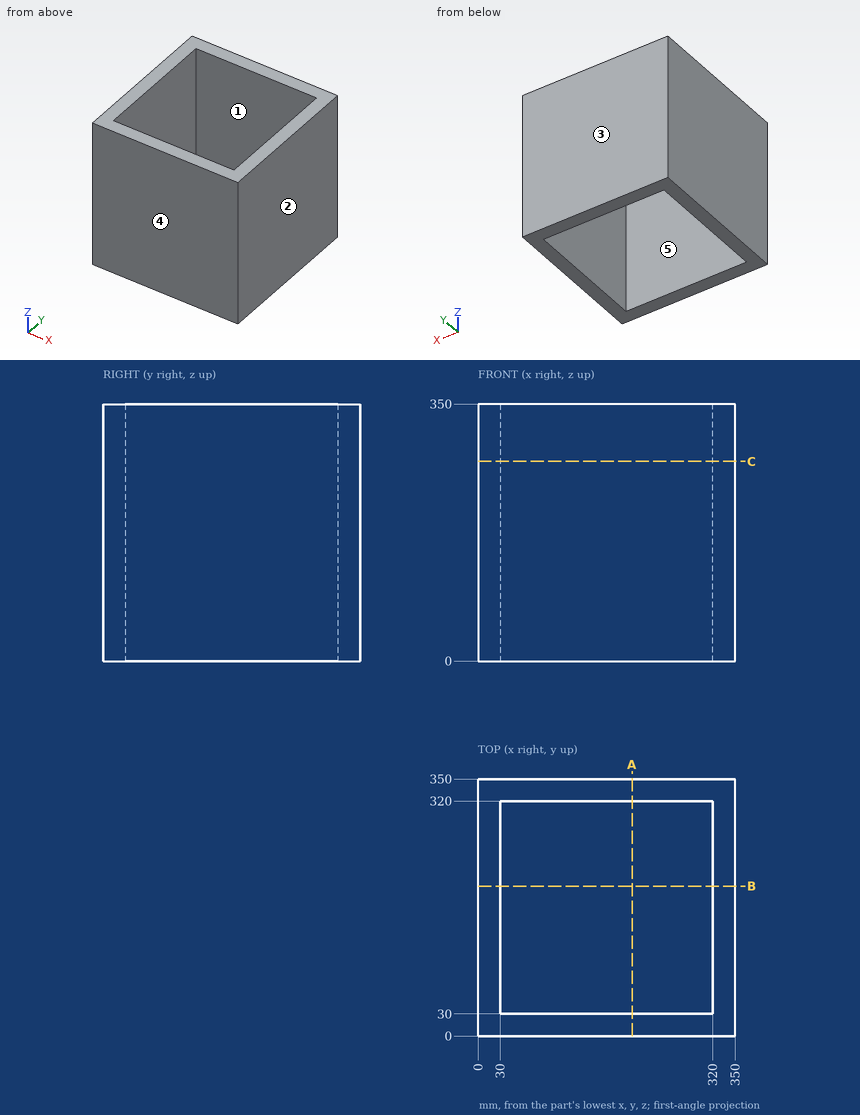
Geometry check sheet. Reference: drawing and pictorial views, mm from the part's lowest x, y, z. A direction names the side the tool comes from. Round coordinates to 2 decimals unless told otherwise and drop trailing zeros. Loops run counter-clockwise (first coordinate to the right, second up) from the corner with the lowest first, then second, coordinate; pieces in that order, holes last. Notation, with made-up numbers: (-7, -3) -> (3, -3) arc R12 cw to (3, 16) -> close; hole circle Ø5 at (68, 25.5). An arc over 180 degrees is marked (long way). Answer as a JSON object with one key per item and string values. Group by question number.
Item 1: Set-up check for the marked faces 4 and 5: record each of +Z, -Z, +X, -X, +Y, -Y from which the full face is reachable in a straight line by a thin tool's end or side.
Item 2: Cross-section at C-C, the plane z = 272. Record the cut outline in (x, y), plus the area to 3 significant figures.
Item 3: Release check for a two-part mould opening along X. For the marked faces 1, 2 and 3 record: pulls with the +X half, pulls with the -X half, needs draft (parallel to the pull), parting line crosses it, or undercut.
Item 4: Thickness scan on line 1 along Y through (x, z) = (242, 178.5). Record the ranges inside material, lowest first.
Item 5: Depth check by flat-ended pin: pin 1 Ø3 at (x, z) = (305.5, 156.5) entering from -Y. Enter the tip coordinate at first touch or a pass-through.
Item 6: Cross-section at A-A, the plane x = 210. Record the cut outline in (y, z), plus the area to 3 significant figures.
Determined:
{
 "1": {"face 4": "+Z, -Z, +X, -X, -Y", "face 5": "+Z, -Z"},
 "2": {"outline": "(0, 0) -> (350, 0) -> (350, 350) -> (0, 350) -> close; hole (30, 30) -> (320, 30) -> (320, 320) -> (30, 320) -> close", "area": "38,400 mm²"},
 "3": {"face 1": "undercut", "face 2": "pulls with the +X half", "face 3": "needs draft"},
 "4": {"line 1": "y = 0 to 30, 320 to 350"},
 "5": {"pin 1": "stops at y = 0"},
 "6": {"outline": "(0, 0) -> (30, 0) -> (30, 350) -> (0, 350) -> close; (320, 0) -> (350, 0) -> (350, 350) -> (320, 350) -> close", "area": "21,000 mm²"}
}
